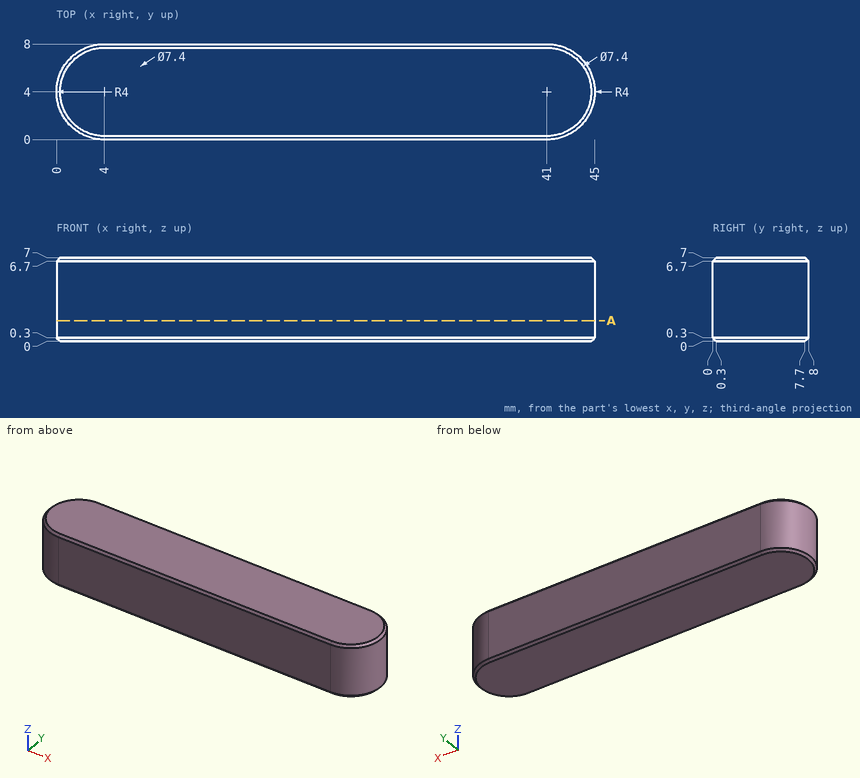
Part print with two shaded views. Sizes in mm from the minimum x, y, z corner. Round coordinates to 2 decimals unless told otherwise and drop trailing zeros. Write each loop counter-clockwise with the first axis right and the second up, starting at its lowest first coordinate (ties: lowest second). Pieces come first, ordered by that corner, then holes. Notation, with made-up numbers: (-12.75, -20) -> (12.25, -20) arc R22 cw to (12.25, 11) -> close; hole circle Ø9 at (3, -38). An arc over 180 degrees is marked (long way). Put each result on its own line as item: value.
Item 1: Slice it at A-A, the plane z = 1.75. Give the cut face in (x, y), plus the area to 3 significant figures.
Here are the results:
outline: (4, 0) -> (41, 0) arc R4 ccw to (41, 8) -> (4, 8) arc R4 ccw to start
area: 346 mm^2
Item 2: Flat gauge pin, fed straight in: P1, Ø4, axis at y = 1.5, z = 2, coming from the -X side. Where does the tip first touch, or does it go through?
Here are the results:
P1: stops at x = 0.03
Item 3: Wall check: probe 1 along X at (y, z) = (5.5, 6.5); probe 2 along X at (y, z) = (1.5, 1.5); probe 3 along Y at (x, z) = (19, 6.75). Give the ranges that are in metal, low to high. Write a range as from..to.
Here are the results:
probe 1: x = 0.29..44.71
probe 2: x = 0.88..44.12
probe 3: y = 0.05..7.95
